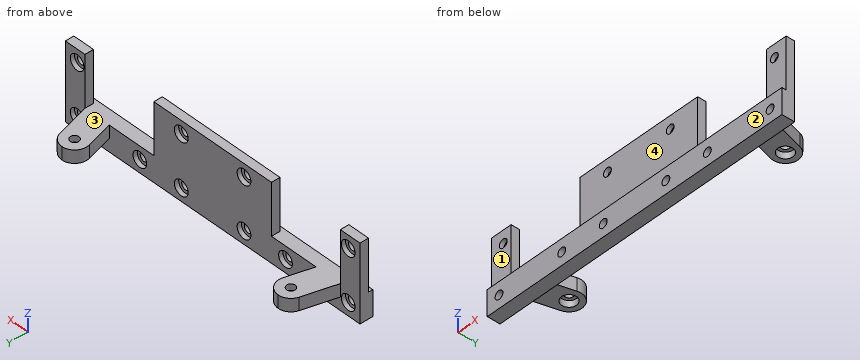
```python
from build123d import *

# Parameters (mm, degrees)
SKETCH_1_R           = 0.75
EXTRUDE_1_DEPTH      = 6
SKETCH_2_R           = 1
CUT_EXTRUDE_1_DEPTH  = 1.5
SKETCH_3_W           = 75.160479418
SKETCH_3_H           = 12
EXTRUDE_2_DEPTH      = 3
SKETCH_4_R           = 0.75
CUT_EXTRUDE_2_DEPTH  = 3
SKETCH_5_W           = 5
SKETCH_5_H           = 12
SKETCH_5_W_2         = 30
CUT_EXTRUDE_3_DEPTH  = 2
SKETCH_6_OUTSIDE_W   = 104.908
SKETCH_6_OUTSIDE_H   = 145.748
SKETCH_6_OUTSIDE_W_2 = 75.160479418
SKETCH_6_OUTSIDE_H_2 = 13
CUT_EXTRUDE_4_DEPTH  = 120.23621269
SKETCH_7_W           = 9
SKETCH_7_H           = 13
CUT_EXTRUDE_5_DEPTH  = 136.845859953
SKETCH_8_R           = 1
CUT_EXTRUDE_6_DEPTH  = 120.122938247
SKETCH_8_3_R         = 1.75
SKETCH_8_3_R_2       = 1
CUT_EXTRUDE_7_DEPTH  = 1.5
SKETCH_9_W           = 5
SKETCH_9_H           = 15
SKETCH_9_W_2         = 30
EXTRUDE_3_DEPTH      = 2
SKETCH_10_W          = 75.160479418
SKETCH_10_H          = 3
EXTRUDE_4_DEPTH      = 3
SKETCH_11_R          = 1
CUT_EXTRUDE_8_DEPTH  = 43.851772619
SKETCH_11_3_R        = 1.75
SKETCH_11_3_R_2      = 1
CUT_EXTRUDE_9_DEPTH  = 1
FILLET_1_R           = 3


with BuildPart() as part:
    # 草图1 → 凸台-拉伸1 (new body)
    with BuildSketch(Plane.XY):
        with BuildLine():
            Line((0, -11.591109915), (26.368582626, -110))
            Line((26.368582626, -110), (32.580239709, -110))
            Line((32.580239709, -110), (2.897777479, 0.776457135))
            ThreePointArc((2.897777479, 0.776457135), (0, 3), (-2.897777479, 0.776457135))
            Line((-2.897777479, 0.776457135), (-32.580239709, -110))
            Line((-32.580239709, -110), (-26.368582626, -110))
            Line((-26.368582626, -110), (0, -11.591109915))
        make_face()
        with Locations((13.665408814, -51)):
            Circle(SKETCH_1_R, mode=Mode.SUBTRACT)
        Circle(SKETCH_1_R, mode=Mode.SUBTRACT)
        with Locations((-13.665408814, -51)):
            Circle(SKETCH_1_R, mode=Mode.SUBTRACT)
    extrude(amount=EXTRUDE_1_DEPTH)

    # 草图2 → 切除-拉伸1 (cut)
    with BuildSketch(Plane(origin=(0, 0, 0), x_dir=(-1, 0, 0), z_dir=(0, 0, -1))):
        Circle(SKETCH_2_R)
        with Locations((13.665408814, -51)):
            Circle(SKETCH_2_R)
        with Locations((-13.665408814, -51)):
            Circle(SKETCH_2_R)
    extrude(amount=-CUT_EXTRUDE_1_DEPTH, mode=Mode.SUBTRACT)

    # 草图3 → 凸台-拉伸2 (add)
    with BuildSketch(Plane.XZ.offset(110)):
        Rectangle(SKETCH_3_W, SKETCH_3_H)
    extrude(amount=EXTRUDE_2_DEPTH)

    # 草图4 → 切除-拉伸2 (cut)
    with BuildSketch(Plane.XY.offset(6)):
        with Locations((-27.59876682, -103)):
            Circle(SKETCH_4_R)
        with Locations((27.59876682, -103)):
            Circle(SKETCH_4_R)
    extrude(amount=-CUT_EXTRUDE_2_DEPTH, mode=Mode.SUBTRACT)

    # 草图5 → 切除-拉伸3 (cut)
    with BuildSketch(Plane(origin=(0, -110, 0), x_dir=(1, 0, 0), z_dir=(0, 1, 0))):
        with Locations((-35.080239709, 0)):
            Rectangle(SKETCH_5_W, SKETCH_5_H)
        with Locations((35.080239709, 0)):
            Rectangle(SKETCH_5_W, SKETCH_5_H)
        Rectangle(SKETCH_5_W_2, SKETCH_5_H)
    extrude(amount=-CUT_EXTRUDE_3_DEPTH, mode=Mode.SUBTRACT)

    # 草图6 outside → 切除-拉伸4 (cut, through all)
    with BuildSketch(Plane(origin=(0, 0, 0), x_dir=(-1, 0, 0), z_dir=(0, 0, -1))):
        with Locations((0, -55)):
            Rectangle(SKETCH_6_OUTSIDE_W, SKETCH_6_OUTSIDE_H)
        with Locations((0, -106.5)):
            Rectangle(SKETCH_6_OUTSIDE_W_2, SKETCH_6_OUTSIDE_H_2, mode=Mode.SUBTRACT)
    extrude(amount=-CUT_EXTRUDE_4_DEPTH, mode=Mode.SUBTRACT)

    # 草图7 → 切除-拉伸5 (cut, through all)
    with BuildSketch(Plane(origin=(37.580239709, 0, 0), x_dir=(0, 0, -1), z_dir=(1, 0, 0))):
        with Locations((1.5, -106.5)):
            Rectangle(SKETCH_7_W, SKETCH_7_H)
    extrude(amount=-CUT_EXTRUDE_5_DEPTH, mode=Mode.SUBTRACT)

    # 草图8 → 切除-拉伸6 (cut, through all)
    with BuildSketch(Plane(origin=(0, 0, 3), x_dir=(-1, 0, 0), z_dir=(0, 0, -1))):
        with Locations(Location((-27.59876682, -103, 0), (0, 0, 90))):
            Circle(SKETCH_8_R)
        with Locations(Location((27.59876682, -103, 0), (0, 0, 90))):
            Circle(SKETCH_8_R)
    extrude(amount=-CUT_EXTRUDE_6_DEPTH, mode=Mode.SUBTRACT)

    # 草图8<3> → 切除-拉伸7 (cut)
    # profile 1 of 2: a face of its own
    with BuildSketch(Plane(origin=(0, 0, 3), x_dir=(-1, 0, 0), z_dir=(0, 0, -1))):
        with Locations(Location((-27.59876682, -103, 0), (0, 0, 90))):
            Circle(SKETCH_8_3_R)
        with Locations(Location((-27.59876682, -103, 0), (0, 0, 90))):
            Circle(SKETCH_8_3_R_2, mode=Mode.SUBTRACT)
    # profile 2 of 2: a face of its own
    with BuildSketch(Plane(origin=(0, 0, 3), x_dir=(-1, 0, 0), z_dir=(0, 0, -1))):
        with Locations(Location((27.59876682, -103, 0), (0, 0, 90))):
            Circle(SKETCH_8_3_R)
        with Locations(Location((27.59876682, -103, 0), (0, 0, 90))):
            Circle(SKETCH_8_3_R_2, mode=Mode.SUBTRACT)
    extrude(amount=-CUT_EXTRUDE_7_DEPTH, mode=Mode.SUBTRACT)

    # 草图9 → 凸台-拉伸3 (add)
    with BuildSketch(Plane(origin=(0, -112, 0), x_dir=(1, 0, 0), z_dir=(0, 1, 0))):
        with Locations((35.080239709, -10.5)):
            Rectangle(SKETCH_9_W, SKETCH_9_H)
        with Locations((0, -10.5)):
            Rectangle(SKETCH_9_W_2, SKETCH_9_H)
        with Locations((-35.080239709, -10.5)):
            Rectangle(SKETCH_9_W, SKETCH_9_H)
    extrude(amount=EXTRUDE_3_DEPTH)

    # 草图10 → 凸台-拉伸4 (add)
    with BuildSketch(Plane(origin=(0, 0, 3), x_dir=(-1, 0, 0), z_dir=(0, 0, -1))):
        with Locations((0, -111.5)):
            Rectangle(SKETCH_10_W, SKETCH_10_H)
    extrude(amount=EXTRUDE_4_DEPTH)

    # 草图11 → 切除-拉伸8 (cut, through all)
    with BuildSketch(Plane(origin=(0, -110, 0), x_dir=(1, 0, 0), z_dir=(0, 1, 0))):
        with Locations(Location((34.580239709, -15, 0), (0, 0, 270))):
            Circle(SKETCH_11_R)
        with Locations(Location((34.580239709, -3, 0), (0, 0, 270))):
            Circle(SKETCH_11_R)
        with Locations(Location((-18.580239709, -3, 0), (0, 0, 270))):
            Circle(SKETCH_11_R)
        with Locations(Location((18.580239709, -3, 0), (0, 0, 270))):
            Circle(SKETCH_11_R)
        with Locations(Location((-34.580239709, -3, 0), (0, 0, 270))):
            Circle(SKETCH_11_R)
        with Locations(Location((-34.580239709, -15, 0), (0, 0, 270))):
            Circle(SKETCH_11_R)
        with Locations((18.580239709, -15)):
            Circle(SKETCH_11_R)
        with Locations((-18.580239709, -15)):
            Circle(SKETCH_11_R)
        with Locations(Location((-8, -3, 0), (0, 0, 270))):
            Circle(SKETCH_11_R)
        with Locations(Location((8, -3, 0), (0, 0, 270))):
            Circle(SKETCH_11_R)
        with Locations(Location((-8, -15, 0), (0, 0, 270))):
            Circle(SKETCH_11_R)
        with Locations(Location((8, -15, 0), (0, 0, 270))):
            Circle(SKETCH_11_R)
    extrude(amount=-CUT_EXTRUDE_8_DEPTH, mode=Mode.SUBTRACT)

    # 草图11<3> → 切除-拉伸9 (cut)
    # profile 1 of 12: a face of its own
    with BuildSketch(Plane(origin=(0, -110, 0), x_dir=(1, 0, 0), z_dir=(0, 1, 0))):
        with Locations(Location((34.580239709, -15, 0), (0, 0, 270))):
            Circle(SKETCH_11_3_R)
        with Locations(Location((34.580239709, -15, 0), (0, 0, 270))):
            Circle(SKETCH_11_3_R_2, mode=Mode.SUBTRACT)
    # profile 2 of 12: a face of its own
    with BuildSketch(Plane(origin=(0, -110, 0), x_dir=(1, 0, 0), z_dir=(0, 1, 0))):
        with Locations(Location((34.580239709, -3, 0), (0, 0, 270))):
            Circle(SKETCH_11_3_R)
        with Locations(Location((34.580239709, -3, 0), (0, 0, 270))):
            Circle(SKETCH_11_3_R_2, mode=Mode.SUBTRACT)
    # profile 3 of 12: a face of its own
    with BuildSketch(Plane(origin=(0, -110, 0), x_dir=(1, 0, 0), z_dir=(0, 1, 0))):
        with Locations(Location((18.580239709, -3, 0), (0, 0, 270))):
            Circle(SKETCH_11_3_R)
        with Locations(Location((18.580239709, -3, 0), (0, 0, 270))):
            Circle(SKETCH_11_3_R_2, mode=Mode.SUBTRACT)
    # profile 4 of 12: a face of its own
    with BuildSketch(Plane(origin=(0, -110, 0), x_dir=(1, 0, 0), z_dir=(0, 1, 0))):
        with Locations(Location((-18.580239709, -3, 0), (0, 0, 270))):
            Circle(SKETCH_11_3_R)
        with Locations(Location((-18.580239709, -3, 0), (0, 0, 270))):
            Circle(SKETCH_11_3_R_2, mode=Mode.SUBTRACT)
    # profile 5 of 12: a face of its own
    with BuildSketch(Plane(origin=(0, -110, 0), x_dir=(1, 0, 0), z_dir=(0, 1, 0))):
        with Locations(Location((-34.580239709, -3, 0), (0, 0, 270))):
            Circle(SKETCH_11_3_R)
        with Locations(Location((-34.580239709, -3, 0), (0, 0, 270))):
            Circle(SKETCH_11_3_R_2, mode=Mode.SUBTRACT)
    # profile 6 of 12: a face of its own
    with BuildSketch(Plane(origin=(0, -110, 0), x_dir=(1, 0, 0), z_dir=(0, 1, 0))):
        with Locations(Location((-34.580239709, -15, 0), (0, 0, 270))):
            Circle(SKETCH_11_3_R)
        with Locations(Location((-34.580239709, -15, 0), (0, 0, 270))):
            Circle(SKETCH_11_3_R_2, mode=Mode.SUBTRACT)
    # profile 7 of 12: a face of its own
    with BuildSketch(Plane(origin=(0, -110, 0), x_dir=(1, 0, 0), z_dir=(0, 1, 0))):
        with Locations((18.580239709, -15)):
            Circle(SKETCH_11_3_R)
        with Locations((18.580239709, -15)):
            Circle(SKETCH_11_3_R_2, mode=Mode.SUBTRACT)
    # profile 8 of 12: a face of its own
    with BuildSketch(Plane(origin=(0, -110, 0), x_dir=(1, 0, 0), z_dir=(0, 1, 0))):
        with Locations((-18.580239709, -15)):
            Circle(SKETCH_11_3_R)
        with Locations((-18.580239709, -15)):
            Circle(SKETCH_11_3_R_2, mode=Mode.SUBTRACT)
    # profile 9 of 12: a face of its own
    with BuildSketch(Plane(origin=(0, -110, 0), x_dir=(1, 0, 0), z_dir=(0, 1, 0))):
        with Locations(Location((-8, -3, 0), (0, 0, 270))):
            Circle(SKETCH_11_3_R)
        with Locations(Location((-8, -3, 0), (0, 0, 270))):
            Circle(SKETCH_11_3_R_2, mode=Mode.SUBTRACT)
    # profile 10 of 12: a face of its own
    with BuildSketch(Plane(origin=(0, -110, 0), x_dir=(1, 0, 0), z_dir=(0, 1, 0))):
        with Locations(Location((8, -3, 0), (0, 0, 270))):
            Circle(SKETCH_11_3_R)
        with Locations(Location((8, -3, 0), (0, 0, 270))):
            Circle(SKETCH_11_3_R_2, mode=Mode.SUBTRACT)
    # profile 11 of 12: a face of its own
    with BuildSketch(Plane(origin=(0, -110, 0), x_dir=(1, 0, 0), z_dir=(0, 1, 0))):
        with Locations(Location((-8, -15, 0), (0, 0, 270))):
            Circle(SKETCH_11_3_R)
        with Locations(Location((-8, -15, 0), (0, 0, 270))):
            Circle(SKETCH_11_3_R_2, mode=Mode.SUBTRACT)
    # profile 12 of 12: a face of its own
    with BuildSketch(Plane(origin=(0, -110, 0), x_dir=(1, 0, 0), z_dir=(0, 1, 0))):
        with Locations(Location((8, -15, 0), (0, 0, 270))):
            Circle(SKETCH_11_3_R)
        with Locations(Location((8, -15, 0), (0, 0, 270))):
            Circle(SKETCH_11_3_R_2, mode=Mode.SUBTRACT)
    extrude(amount=-CUT_EXTRUDE_9_DEPTH, mode=Mode.SUBTRACT)

    # 圆角1
    fillet_1_edges = [part.edges().sort_by_distance(p)[0] for p in [
        (-29.900747784, -100, 4.5),
        (-23.689090702, -100, 4.5),
        (23.689090702, -100, 4.5),
        (29.900747784, -100, 4.5),
    ]]
    fillet(fillet_1_edges, radius=FILLET_1_R - 0.0001)  # a hair under: the kernel refuses the full size


solid = part.part
```
Can you work these out from the model? Positions are in its coordinate system, mm. Face numbers are marked on the shaded views. A direction names the side the tool comes from. Round coordinates to 2 decimals unless told otherwise and drop trailing zeros. Loops run counter-clockwise (first coordinate to the right, second up) from the corner with the lowest first, then second, coordinate; pieces in that order, holes last. Notation, with made-up numbers: (87.25, -25) -> (114.25, -25) arc R19 cw to (114.25, -19) -> close; hole circle Ø1 at (-37, 48). An arc over 180 degrees is marked (long way). One line per item, written item: value. Start each with the question number.
1. If we mould it in two halves opening along X, with no side actions, what happens to the marked faces 3 and 4? For each: pulls with the +X half, pulls with the -X half, needs draft (parallel to the pull), parting line crosses it, or undercut.
2. If we section it at C-C, the plane y = -103: Write out the boundary of the cut face in (x, z).
3. If I drill on probe 1 along Y at (x, z) = (17.5, 2.25); probe 2 along Y at (x, z) = (-5, 5.75); probe 3 along Z at (x, y) = (-21.5, -111), over which ranges is the centre line in solid material (lowest first)?
4. For the marked faces 1 and 2, which set-ups out of +Z, -Z, +X, -X, +Y, -Y let a thin tool reach every point of the face, with its end or its side?
5. If we section it at B-B, the plane z = 11: Write out the boundary of the cut face in (x, y), then the cut area to 3 significant figures.
6. For pin 1 (3 mm diameter, centred on x = -34.5, z = 15.5, fed in from +Y); pin 2 (1.2 mm diameter, centred on x = 34.58, z = 3, fed in from +Y); pin 3 (2 mm diameter, centred on x = 0.5, z = 10, fed in from -Y); pin 4 (1 mm diameter, centred on x = -19, z = 4, fed in from +Y), each with a flat end and sliding along its axis, tell me the tip position at first contact or that it passes through.
7. If we section it at D-D, the plane z = 15: Give the number of separate pieces and of enclosed holes in the cut face, then the cut area to 3 significant figures.
8. If we section it at A-A, the plane x = -8: Write out the boundary of the cut face in (y, z), then the cut area to 3 significant figures.
Calculated:
1. face 3: undercut
1. face 4: needs draft
2. outline: (-30.7, 3) -> (-29.35, 3) -> (-29.35, 4.5) -> (-28.6, 4.5) -> (-28.6, 6) -> (-30.7, 6) -> close; (-26.6, 4.5) -> (-25.85, 4.5) -> (-25.85, 3) -> (-24.6, 3) -> (-24.6, 6) -> (-26.6, 6) -> close; (24.6, 3) -> (25.85, 3) -> (25.85, 4.5) -> (26.6, 4.5) -> (26.6, 6) -> (24.6, 6) -> close; (28.6, 4.5) -> (29.35, 4.5) -> (29.35, 3) -> (30.7, 3) -> (30.7, 6) -> (28.6, 6) -> close
3. probe 1: y = -113 to -111
3. probe 2: y = -113 to -110
3. probe 3: z = 0 to 6
4. face 1: +Z, +X, -X, -Y
4. face 2: +Z, -Z, +X, -X, -Y
5. outline: (-37.58, -112) -> (-32.58, -112) -> (-32.58, -110) -> (-37.58, -110) -> close; (-15, -112) -> (15, -112) -> (15, -110) -> (-15, -110) -> close; (32.58, -112) -> (37.58, -112) -> (37.58, -110) -> (32.58, -110) -> close
5. area: 80.0 mm²
6. pin 1: stops at y = -110
6. pin 2: passes through
6. pin 3: stops at y = -112
6. pin 4: stops at y = -111
7. separate pieces: 7
7. enclosed holes: 0
7. area: 58.0 mm²
8. outline: (-113, 0) -> (-110, 0) -> (-110, 1.25) -> (-111, 1.25) -> (-111, 2) -> (-113, 2) -> close; (-113, 4) -> (-111, 4) -> (-111, 4.75) -> (-110, 4.75) -> (-110, 13.25) -> (-111, 13.25) -> (-111, 14) -> (-112, 14) -> (-112, 6) -> (-113, 6) -> close; (-112, 16) -> (-111, 16) -> (-111, 16.75) -> (-110, 16.75) -> (-110, 18) -> (-112, 18) -> close
8. area: 29.0 mm²
